Geometry: final body of the model. Coordinates: model frame, mm. Face numbers are marked on the shaded views. A direction names the side the tool comes from. Give positions to 0.01 mm unless a question says otherwise; leave off trailing zeros. Order: outer loops, then holes, each group sorted by start corner. A loop starts at its lowest first (then second) coordinate and runs counter-clockwise, first axis right, second up. Notation, with made-up numbers: (-39, 67) - (-13, 67) arc R9 ccw to (-13, 78) - close; hole circle Ø6 at (40.5, -36.5). An arc over 180 degrees is marked (long way). Use one line per item in the form item = value.
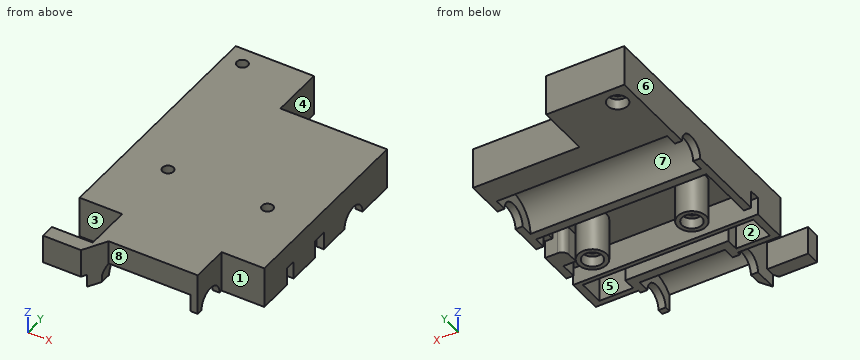
from build123d import *

# Parameters (mm, degrees)
CROQUIS1_W              = 52
CROQUIS1_H              = 90
SALIENTE_EXTRUIR1_DEPTH = 11.6
CORTAR_EXTRUIR1_DEPTH   = 48
CORTAR_EXTRUIR2_DEPTH   = 24
CORTAR_EXTRUIR3_DEPTH   = 53
CORTAR_EXTRUIR4_DEPTH   = 53
CORTAR_EXTRUIR7_DEPTH   = 8
CROQUIS7_R              = 4
SALIENTE_EXTRUIR2_DEPTH = 12
CROQUIS8_W              = 2
CROQUIS8_H              = 4
CORTAR_EXTRUIR8_DEPTH   = 5
SALIENTE_EXTRUIR4_DEPTH = 8
CROQUIS10_R             = 1.55
CORTAR_EXTRUIR9_DEPTH   = 16.6
CROQUIS11_R             = 2.8
CROQUIS11_R_2           = 1.55
CORTAR_EXTRUIR10_DEPTH  = 3
CROQUIS12_W             = 5
CROQUIS12_H             = 3
CORTAR_EXTRUIR11_DEPTH  = 53
CROQUIS13_W             = 30
CROQUIS13_H             = 15
CORTAR_EXTRUIR12_DEPTH  = 12
CROQUIS14_R             = 1.55
CORTAR_EXTRUIR13_DEPTH  = 12
CROQUIS14_3_R           = 2.8
CROQUIS14_3_R_2         = 1.55
CORTAR_EXTRUIR14_DEPTH  = 3
CROQUIS15_W             = 48
CROQUIS15_H             = 1.2
SALIENTE_EXTRUIR5_DEPTH = 8
CROQUIS16_W             = 12
CROQUIS16_H             = 20
CORTAR_EXTRUIR15_DEPTH  = 12.6
CROQUIS17_W             = 12
CROQUIS17_H             = 20
CORTAR_EXTRUIR16_DEPTH  = 12.6
CROQUIS18_W             = 11.5
CROQUIS18_H             = 4
SALIENTE_EXTRUIR6_DEPTH = 8
CROQUIS19_R             = 4
SALIENTE_EXTRUIR7_DEPTH = 12
CROQUIS20_R             = 1.55
CORTAR_EXTRUIR17_DEPTH  = 16.6
CROQUIS20_3_R           = 2.8
CROQUIS20_3_R_2         = 1.55
CORTAR_EXTRUIR18_DEPTH  = 3
CROQUIS21_W             = 28
CROQUIS21_H             = 2.8
CORTAR_EXTRUIR19_DEPTH  = 16.6
CORTAR_EXTRUIR20_DEPTH  = 16.6


with BuildPart() as part:
    # Croquis1 → Saliente-Extruir1 (new body)
    with BuildSketch(Plane.XY):
        with Locations((26, 45)):
            Rectangle(CROQUIS1_W, CROQUIS1_H)
    extrude(amount=SALIENTE_EXTRUIR1_DEPTH)

    # Croquis2 → Cortar-Extruir1 (cut)
    with BuildSketch(Plane(origin=(50, 0, 0), x_dir=(0, 0, -1), z_dir=(1, 0, 0))):
        with BuildLine():
            Line((0, 52.45), (0, 67.55))
            ThreePointArc((0, 67.55), (-7.55, 60), (0, 52.45))
        make_face()
    extrude(amount=-CORTAR_EXTRUIR1_DEPTH, mode=Mode.SUBTRACT)

    # Croquis3 → Cortar-Extruir2 (cut)
    with BuildSketch(Plane(origin=(38, 0, 0), x_dir=(0, 0, -1), z_dir=(1, 0, 0))):
        with BuildLine():
            Line((0, 7.45), (0, 22.55))
            ThreePointArc((0, 22.55), (-7.55, 15), (0, 7.45))
        make_face()
    extrude(amount=-CORTAR_EXTRUIR2_DEPTH, mode=Mode.SUBTRACT)

    # Croquis4 → Cortar-Extruir3 (cut, through all)
    with BuildSketch(Plane(origin=(52, 0, 0), x_dir=(0, 0, -1), z_dir=(1, 0, 0))):
        with BuildLine():
            ThreePointArc((0, 64.05), (-4.05, 60), (0, 55.95))
            Line((0, 55.95), (0, 64.05))
        make_face()
        with BuildLine():
            Line((0, 64.05), (0, 55.95))
            ThreePointArc((0, 55.95), (2.863782464, 57.136217536), (4.05, 60))
            ThreePointArc((4.05, 60), (2.863782464, 62.863782464), (0, 64.05))
        make_face()
    extrude(amount=-CORTAR_EXTRUIR3_DEPTH, mode=Mode.SUBTRACT)

    # Croquis5 → Cortar-Extruir4 (cut, through all)
    with BuildSketch(Plane(origin=(52, 0, 0), x_dir=(0, 0, -1), z_dir=(1, 0, 0))):
        with BuildLine():
            ThreePointArc((0, 19.05), (-4.05, 15), (0, 10.95))
            Line((0, 10.95), (0, 19.05))
        make_face()
        with BuildLine():
            Line((0, 19.05), (0, 10.95))
            ThreePointArc((0, 10.95), (2.863782464, 12.136217536), (4.05, 15))
            ThreePointArc((4.05, 15), (2.863782464, 17.863782464), (0, 19.05))
        make_face()
    extrude(amount=-CORTAR_EXTRUIR4_DEPTH, mode=Mode.SUBTRACT)

    # Croquis6 → Cortar-Extruir7 (cut)
    with BuildSketch(Plane(origin=(0, 0, 0), x_dir=(-1, 0, 0), z_dir=(0, 0, -1))):
        Polygon((-2, 49.95), (-2, 21.55), (-11.5, 21.55), (-11.5, 25.05), (-40.5, 25.05), (-40.5, 21.55), (-50, 21.55), (-50, 49.95), align=None)
    extrude(amount=-CORTAR_EXTRUIR7_DEPTH, mode=Mode.SUBTRACT)

    # Croquis7 → Saliente-Extruir2 (add)
    with BuildSketch(Plane(origin=(0, 0, 8), x_dir=(-1, 0, 0), z_dir=(0, 0, -1))):
        with Locations((-40, 40.55)):
            Circle(CROQUIS7_R)
    extrude(amount=SALIENTE_EXTRUIR2_DEPTH)

    # Croquis8 → Cortar-Extruir8 (cut)
    with BuildSketch(Plane(origin=(0, 0, 0), x_dir=(-1, 0, 0), z_dir=(0, 0, -1))):
        with Locations((-51, 44.65)):
            Rectangle(CROQUIS8_W, CROQUIS8_H)
    extrude(amount=-CORTAR_EXTRUIR8_DEPTH, mode=Mode.SUBTRACT)

    # Croquis9 → Saliente-Extruir4 (add)
    with BuildSketch(Plane(origin=(0, 0, 0), x_dir=(-1, 0, 0), z_dir=(0, 0, -1))):
        with BuildLine():
            Line((-52, 42.65), (-48.495265185, 42.65))
            ThreePointArc((-48.495265185, 42.65), (-47.081051623, 42.064213562), (-46.495265185, 40.65))
            Line((-46.495265185, 40.65), (-46.495265185, 37.65))
            Line((-46.495265185, 37.65), (-52, 37.65))
            Line((-52, 37.65), (-52, 42.65))
        make_face()
    extrude(amount=-SALIENTE_EXTRUIR4_DEPTH)

    # Croquis10 → Cortar-Extruir9 (cut, through all)
    with BuildSketch(Plane(origin=(0, 0, -4), x_dir=(-1, 0, 0), z_dir=(0, 0, -1))):
        with Locations((-40, 40.55)):
            Circle(CROQUIS10_R)
    extrude(amount=-CORTAR_EXTRUIR9_DEPTH, mode=Mode.SUBTRACT)

    # Croquis11 → Cortar-Extruir10 (cut)
    with BuildSketch(Plane(origin=(0, 0, -4), x_dir=(-1, 0, 0), z_dir=(0, 0, -1))):
        with Locations((-40, 40.55)):
            Circle(CROQUIS11_R)
        with Locations((-40, 40.55)):
            Circle(CROQUIS11_R_2, mode=Mode.SUBTRACT)
    extrude(amount=-CORTAR_EXTRUIR10_DEPTH, mode=Mode.SUBTRACT)

    # Croquis12 → Cortar-Extruir11 (cut, through all)
    with BuildSketch(Plane(origin=(52, 0, 0), x_dir=(0, 0, -1), z_dir=(1, 0, 0))):
        with Locations((-2.5, 31.65)):
            Rectangle(CROQUIS12_W, CROQUIS12_H)
    extrude(amount=-CORTAR_EXTRUIR11_DEPTH, mode=Mode.SUBTRACT)

    # Croquis13 → Cortar-Extruir12 (cut)
    with BuildSketch(Plane(origin=(0, 0, 0), x_dir=(-1, 0, 0), z_dir=(0, 0, -1))):
        with Locations((-37, 82.5)):
            Rectangle(CROQUIS13_W, CROQUIS13_H)
    extrude(amount=-CORTAR_EXTRUIR12_DEPTH, mode=Mode.SUBTRACT)

    # Croquis14 → Cortar-Extruir13 (cut)
    with BuildSketch(Plane(origin=(0, 0, 0), x_dir=(-1, 0, 0), z_dir=(0, 0, -1))):
        with Locations((-5, 85)):
            Circle(CROQUIS14_R)
    extrude(amount=-CORTAR_EXTRUIR13_DEPTH, mode=Mode.SUBTRACT)

    # Croquis14<3> → Cortar-Extruir14 (cut)
    with BuildSketch(Plane(origin=(0, 0, 0), x_dir=(-1, 0, 0), z_dir=(0, 0, -1))):
        with Locations((-5, 85)):
            Circle(CROQUIS14_3_R)
        with Locations((-5, 85)):
            Circle(CROQUIS14_3_R_2, mode=Mode.SUBTRACT)
    extrude(amount=-CORTAR_EXTRUIR14_DEPTH, mode=Mode.SUBTRACT)

    # Croquis15 → Saliente-Extruir5 (add)
    with BuildSketch(Plane(origin=(0, 0, 8), x_dir=(-1, 0, 0), z_dir=(0, 0, -1))):
        with Locations((-26, 29.55)):
            Rectangle(CROQUIS15_W, CROQUIS15_H)
    extrude(amount=SALIENTE_EXTRUIR5_DEPTH)

    # Croquis16 → Cortar-Extruir15 (cut, through all)
    with BuildSketch(Plane(origin=(0, 0, 0), x_dir=(-1, 0, 0), z_dir=(0, 0, -1))):
        with Locations((-46, 10)):
            Rectangle(CROQUIS16_W, CROQUIS16_H)
    extrude(amount=-CORTAR_EXTRUIR15_DEPTH, mode=Mode.SUBTRACT)

    # Croquis17 → Cortar-Extruir16 (cut, through all)
    with BuildSketch(Plane(origin=(0, 0, 0), x_dir=(-1, 0, 0), z_dir=(0, 0, -1))):
        with Locations((-6, 10)):
            Rectangle(CROQUIS17_W, CROQUIS17_H)
    extrude(amount=-CORTAR_EXTRUIR16_DEPTH, mode=Mode.SUBTRACT)

    # Croquis18 → Saliente-Extruir6 (add)
    with BuildSketch(Plane.XY.offset(11.6)):
        with Locations((6.25, 4.8)):
            Rectangle(CROQUIS18_W, CROQUIS18_H)
    extrude(amount=-SALIENTE_EXTRUIR6_DEPTH)

    # Croquis19 → Saliente-Extruir7 (add)
    with BuildSketch(Plane(origin=(0, 0, 8), x_dir=(-1, 0, 0), z_dir=(0, 0, -1))):
        with Locations((-12, 40.55)):
            Circle(CROQUIS19_R)
    extrude(amount=SALIENTE_EXTRUIR7_DEPTH)

    # Croquis20 → Cortar-Extruir17 (cut, through all)
    with BuildSketch(Plane(origin=(0, 0, -4), x_dir=(-1, 0, 0), z_dir=(0, 0, -1))):
        with Locations((-12, 40.55)):
            Circle(CROQUIS20_R)
    extrude(amount=-CORTAR_EXTRUIR17_DEPTH, mode=Mode.SUBTRACT)

    # Croquis20<3> → Cortar-Extruir18 (cut)
    with BuildSketch(Plane(origin=(0, 0, -4), x_dir=(-1, 0, 0), z_dir=(0, 0, -1))):
        with Locations((-12, 40.55)):
            Circle(CROQUIS20_3_R)
        with Locations((-12, 40.55)):
            Circle(CROQUIS20_3_R_2, mode=Mode.SUBTRACT)
    extrude(amount=-CORTAR_EXTRUIR18_DEPTH, mode=Mode.SUBTRACT)

    # Croquis21 → Cortar-Extruir19 (cut, through all)
    with BuildSketch(Plane.XY.offset(11.6)):
        with Locations((26, 1.4)):
            Rectangle(CROQUIS21_W, CROQUIS21_H)
    extrude(amount=-CORTAR_EXTRUIR19_DEPTH, mode=Mode.SUBTRACT)

    # Croquis22 → Cortar-Extruir20 (cut, through all)
    with BuildSketch(Plane.XY.offset(11.6)):
        Polygon((11.184549083, 2.8), (40, 2.8), (40, 9.264101615), (14.916599891, 9.264101615), align=None)
    extrude(amount=-CORTAR_EXTRUIR20_DEPTH, mode=Mode.SUBTRACT)


solid = part.part
(1) Ray query, line 1 along X through (y, z) = (24.5, 2.25); line 2 along Y through (x, z) = (20, 3.5); line 3 along Y through (x, z) = (26, 5.25). Return the intervals inside material, ascending.
Computed values:
line_1 = 0 to 2, 11.5 to 40.5, 50 to 52
line_2 = 21.69 to 25.05, 28.95 to 30.15, 49.95 to 53.31, 66.69 to 90
line_3 = 9.26 to 9.57, 20.43 to 25.05, 28.95 to 30.15, 49.95 to 54.57, 65.43 to 75
(2) Pull-direction query (Y, two-part tool) for the marked faces 5, 6, 7 and 8; classes: released by +Y, released by -Y, zero draft, split by the parting line, or undercut.
Computed values:
face_5 = undercut
face_6 = zero draft
face_7 = undercut
face_8 = released by -Y
(3) Cut plane C-C on y = 60. Output: boundary loops of the cut face in (x, z).
Computed values:
outline = (0, 4.05) - (2, 4.05) - (2, 7.55) - (50, 7.55) - (50, 4.05) - (52, 4.05) - (52, 11.6) - (0, 11.6) - close
(4) Cut plane D-D on z = 6.5. Give the number of separate pieces and of enclosed holes in the cut face, plus the area to 3 significant figures.
Computed values:
separate_pieces = 3
enclosed_holes = 7
area = 1,880 mm²
(5) Contact query for flat-ended pins moving along their axis: pin 1 Ø8 at (y, z) = (47, 2.5) entering from -X; pin 2 Ø3 at (x, z) = (39.5, 6) entering from +Y; pin 3 Ø2 at (x, z) = (26, 9) entering from -Y; pin 4 Ø2 at (x, y) = (18.5, 35.5) entering from -Z. Output: stop coordinate, or through.
Computed values:
pin_1 = 0
pin_2 = 75
pin_3 = 9.26
pin_4 = 8
(6) Cut plane B-B on x = 5. Output: boundary loops of the cut face in (y, z).
Computed values:
outline = (2.8, 3.6) - (6.8, 3.6) - (6.8, 11.6) - (2.8, 11.6) - close; (20, 0) - (21.55, 0) - (21.55, 8) - (28.95, 8) - (28.95, 0) - (30.15, 0) - (30.15, 8) - (49.95, 8) - (49.95, 0) - (52.45, 0) arc R7.55 cw to (67.55, 0) - (82.2, 0) - (82.2, 3) - (83.45, 3) - (83.45, 11.6) - (20, 11.6) - close; (86.55, 3) - (87.8, 3) - (87.8, 0) - (90, 0) - (90, 11.6) - (86.55, 11.6) - close
(7) Cut plane A-A on y = 85. Output: boundary loops of the cut face in (x, z), plus the area to 3 significant figures.
Computed values:
outline = (0, 0) - (2.2, 0) - (2.2, 3) - (3.45, 3) - (3.45, 11.6) - (0, 11.6) - close; (6.55, 3) - (7.8, 3) - (7.8, 0) - (22, 0) - (22, 11.6) - (6.55, 11.6) - close
area = 212 mm²
(8) Reachability of the marked faces 1, 2, 3 and 4 from +Z, -Z, +X, -X, +Y, -Y: full face, straight path, thin tool, end or side. Return the list, or none.
Computed values:
face_1 = +Z, -Z, +X, -Y
face_2 = -Z
face_3 = +Z, -Z, -X
face_4 = +Z, -Z, +X, +Y
